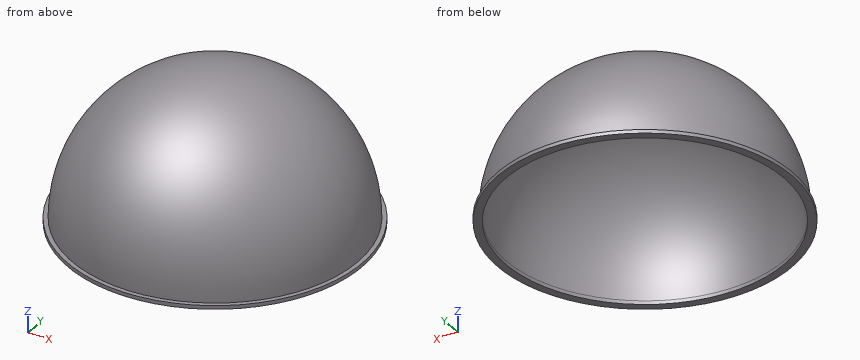
from build123d import *

# Parameters (mm, degrees)
SHELL1_T            = -2
SKETCH2_R           = 81.25
SKETCH2_R_2         = 76.85
BOSS_EXTRUDE1_DEPTH = 2


# Read off the part's stored shape, not the designer's step: Revolve1
with BuildPart() as part:
    # Revolve1 outline → Revolve1 (revolve)
    with BuildSketch(Plane.XZ):
        with BuildLine():
            Line((0, 0), (78.85, -7.9e-08))
            ThreePointArc((78.85, -7.9e-08), (55.755369724, 55.755369669), (0, 78.85))
            Line((0, 78.85), (0, 0))
        make_face()
    revolve(axis=Axis((0, 0, 0), (0, 0, 1)))

    # Shell1
    shell1_openings = [part.faces().sort_by_distance(p)[0] for p in [
        (0, 0, 0),
    ]]
    offset(amount=SHELL1_T, openings=shell1_openings, kind=Kind.INTERSECTION)

    # Sketch2 → Boss-Extrude1 (add)
    with BuildSketch(Plane(origin=(0, 0, 0), x_dir=(-1, 0, 0), z_dir=(0, 0, -1))):
        Circle(SKETCH2_R)
        Circle(SKETCH2_R_2, mode=Mode.SUBTRACT)
    extrude(amount=BOSS_EXTRUDE1_DEPTH)


solid = part.part
Geometry check sheet. Reference: the model listing, model coordinates, mm. Coordinates: 2 decimals unless noted, no trailing zeros. Order: outer loops, then holes, each group sorted by start corner. A loop starts at its lowest first (then second) coordinate and runs counter-clockwise, first axis right, second up. Notation, with made-up numbers: (60, 10) - (112, 10) arc R29 ccw to (112, 30) - close; hole circle Ø9 at (67, -15). An arc over 180 degrees is marked (long way). One line per item, written item: value.
(1) Thickness scan on probe 1 along Y at (x, z) = (0, -0.45); probe 2 along X at (y, z) = (-38, 55); probe 3 along X at (y, z) = (-28, 41.5). Record the ranges inside material, lowest first. Write a range as from..to.
Data:
probe 1: y = -81.25..-76.85, 76.85..81.25
probe 2: x = -41.81..-37.91, 37.91..41.81
probe 3: x = -60.92..-58.31, 58.31..60.92
(2) Sectioned sample at A-A (y = 0). Enter the section's corners in (x, z).
Data:
outline: (-81.25, -2) - (-76.85, -2) - (-76.85, 0) arc R76.85 cw to (76.85, 0) - (76.85, -2) - (81.25, -2) - (81.25, 0) - (78.85, 0) arc R78.85 ccw to (-78.85, 0) - (-81.25, 0) - close
(3) Depth check by flat-ended pin: pin 1 Ø8 at (x, z) = (0, 30) entering from +Y; pin 2 Ø5 at (x, z) = (-32.5, 34) entering from -Y; pin 3 Ø1.5 at (x, y) = (8, 12.5) entering from +Z. Enter the tip coordinate at first touch or a pass-through.
Data:
pin 1: stops at y = 74.44
pin 2: stops at y = -65.07
pin 3: stops at z = 77.58
(4) Sectioned sample at C-C (z = 9.5). Enter the section's corners in (x, y), and give its area (3 significant figures).
Data:
outline: circle Ø156.55 at (0, 0); hole circle Ø152.52 at (0, 0)
area: 978 mm^2
